Study the drawing (mm; zero at the part's minimum x, y, z) and answer. Give positions to 0.01 mm unless a question says otherwise; leave off trailing zeros. Order: outer loops, then holes, each group sorted by start corner. A loop starts at its lowest first (then second) coordinate and runs counter-clockwise, first axis right, second up.
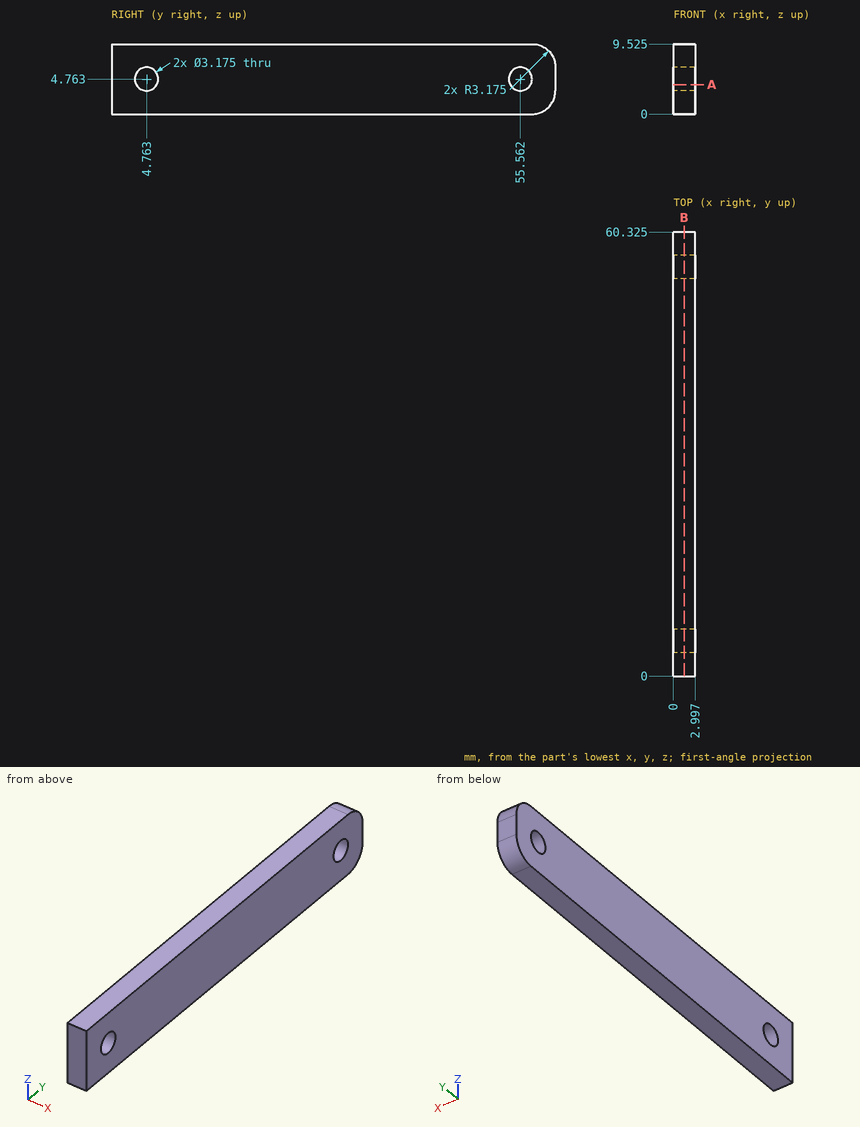
1) Given P1, Ø3, axis at y = 55.56, z = 4.76, coming from the -X side, flat-ended and moving along its own axis, determine where the tip first touches the part or whether it passes through.
Geometry says:
P1: passes through
2) Straight lines are drawn through the part: probe 1 along Y at (x, z) = (0.25, 4) (1 decimal); probe 2 along Y at (x, z) = (2.8, 5.75) (1 decimal); probe 3 along Y at (x, z) = (1.3, 6.5). For each, find the intervals that lie inside material, in ascending order.
Geometry says:
probe 1: y = 0 to 3.4, 6.2 to 54.2, 57 to 60.3
probe 2: y = 0 to 3.5, 6 to 54.3, 56.8 to 60.3
probe 3: y = 0 to 60.32
3) Find section A-A (z = 4). Write down the section's boundary in (x, y) (1 decimal), then the cut area to 3 significant figures.
Geometry says:
outline: (0, 0) - (3, 0) - (3, 3.4) - (0, 3.4) - close; (0, 6.2) - (3, 6.2) - (3, 54.2) - (0, 54.2) - close; (0, 57) - (3, 57) - (3, 60.3) - (0, 60.3) - close
area: 164 mm2
4) Find section B-B (x = 1.45). Count the separate pieces of the cut face and the enclosed holes in it.
Geometry says:
separate pieces: 1
enclosed holes: 2
